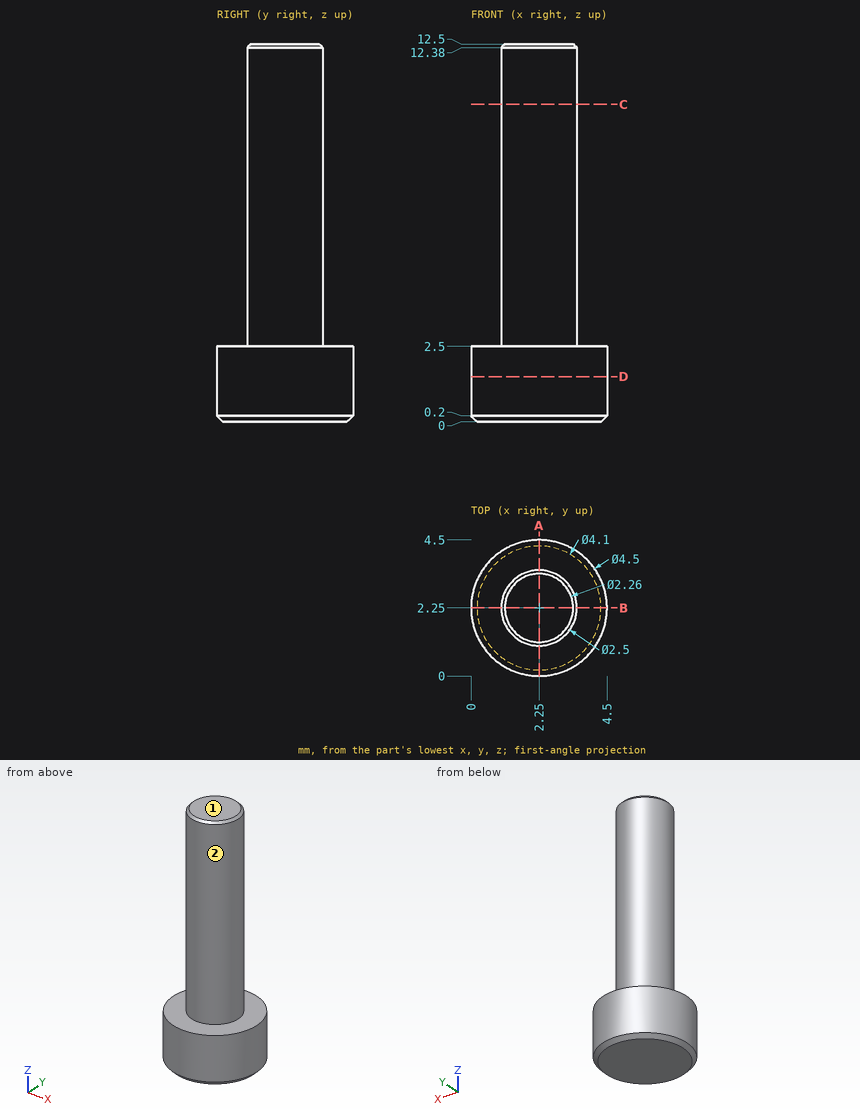
Geometry check sheet. Reference: drawing and pictorial views, mm from the part's lowest x, y, z. A direction names the side the tool comes from. Coordinates: 2 decimals unless noted, no trailing zeros. Order: outer loops, then holes, each group sorted by start corner. A loop starts at its lowest first (then second) coordinate and runs counter-clockwise, first axis right, second up. Notation, with made-up numbers: (-22, 20) -> (8, 20) arc R35 ccw to (8, 54) -> close; hole circle Ø7 at (17, -21.75). An arc over 180 degrees is marked (long way). Use CSV: the item, a comma, the result in double quotes. Start each with the question number.
Q1. Depth check by flat-ended pin: P1, Ø2, axis at y = 1.5, z = 8, coming from the -X side. Enter the tip coordinate at first touch or a pass-through.
Q2. Tool access check on the marked faces 1 and 2. Record the directions out of +Z, -Z, +X, -X, +Y, -Y that give a thin tool (end or side, any length) a straight path to the whole face; none if there is none.
Q3. Thickness scan on line 1 along X through (y, z) = (2.35, 1); line 2 along Z through (x, y) = (3.8, 1.9); line 3 along Z through (x, y) = (1.75, 4.35). Record the ranges inside material, lowest first.
Q4. Section check D-D, the plane z = 1.5. Record the cut outline in (x, y), and give its area (3 significant figures).
Q5. Section check A-A, the plane x = 2.25. Record the cut outline in (y, z).
Q6. Section check C-C, the plane z = 10.5. Record the cut outline in (x, y), and give its area (3 significant figures).
Returned:
1,P1,"stops at x = 1"
2,face 1,"+Z, +X, -X, +Y, -Y"
2,face 2,"+Z"
3,line 1,"x = 0 to 4.5"
3,line 2,"z = 0 to 2.5"
3,line 3,"z = 0.11 to 2.5"
4,outline,"circle Ø4.5 at (2.25, 2.25)"
4,area,"15.9 mm^2"
5,outline,"(0, 0.2) -> (0.2, 0) -> (4.3, 0) -> (4.5, 0.2) -> (4.5, 2.5) -> (3.5, 2.5) -> (3.5, 12.38) -> (3.38, 12.5) -> (1.12, 12.5) -> (1, 12.38) -> (1, 2.5) -> (0, 2.5) -> close"
6,outline,"circle Ø2.5 at (2.25, 2.25)"
6,area,"4.91 mm^2"
